The listing builds one solid part. Answer for the finished solid, in the listing's coordinates (mm). Face numbers are marked on the shaded views. A direction names the side the tool comes from. Round coordinates to 2 decimals unless told otherwise and drop trailing zeros. Order: outer loops, then holes, each group sorted by start corner. A loop starts at its lowest first (then second) coordinate and runs counter-clockwise, first axis right, second up. Notation, with made-up numbers: M -1.75,-37.5 L 23.25,-37.5 A24 cw 23.25,-26.5 Z; hole C 89.25,61.5 d4. An arc over 180 degrees is marked long. Write item = value, one per line. Start each with the question number.
(1) A cutting plane is placed at C-C, the plane x = 88.5. Determine the outline of the cut face in (y, z).
(2) For a pull along Z with two mould halves and no side action, classify the marked faces 1, 2, 3 and 4 as released by +Z, released by -Z, zero draft, split by the parting line, or undercut.
(3) A cutting plane is placed at B-B, the plane z = -24. Determine the outline of the cut face in (x, y), and give its area (3 significant figures).
(4) Straight lines are drawn through the part: probe 1 along Y at (x, z) = (230.5, -46); probe 2 along Z at (x, y) = (256, 197). For each, find the intervals that lie inside material, in ascending order. Write a range as from..to.
(5) A cutting plane is placed at A-A, the plane y = 224. Determine the outline of the cut face in (x, z), and give its area (3 significant figures).
(6) Which of the six approach directions +Z, -Z, +X, -X, +Y, -Y give full straight-line access (tool end or side, diameter ignored) to the marked faces 5 and 6?
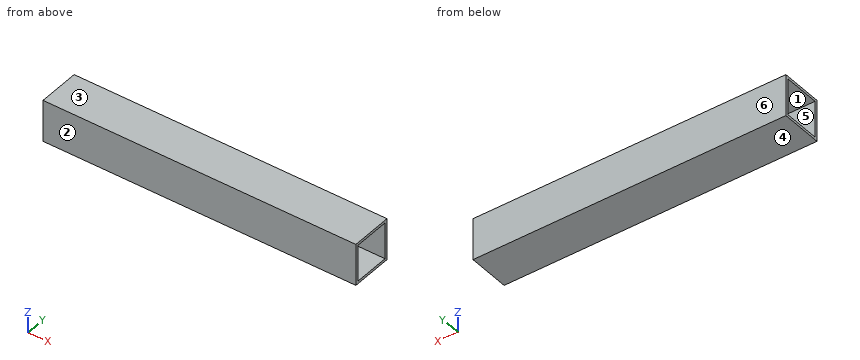
Solid Edge part; units mm, degrees
sketch "Sketch1" plane through (0, 0, 0) normal (1, 0, 0) x (0, 1, 0)
  line L0 (250, 0) -> (250, -80)
  line L1 (250, -80) -> (170, -80)
  line L2 (170, 0) -> (170, -80)
  line L3 (250, 0) -> (170, 0)
extrude "Protrusion1" add sketch "Sketch1" against normal up to vertex (250 mm away) and the other way up to vertex (350 mm away)
sketch "Sketch2" plane through (-250, 210, -40) normal (-1, 0, 0) x (0, -1, 0)
  line L0 (-35, 35) -> (-35, -35)
  line L1 (-35, -35) -> (35, -35)
  line L2 (35, -35) -> (35, 35)
  line L3 (35, 35) -> (-35, 35)
extrude "Cutout1" cut sketch "Sketch2" against normal through all
properties material "Fe360"
Reported:
q1.outline = M 170,-80 L 250,-80 L 250,0 L 170,0 Z; hole M 175,-75 L 245,-75 L 245,-5 L 175,-5 Z
q2.face_1 = undercut
q2.face_2 = zero draft
q2.face_3 = released by +Z
q2.face_4 = released by -Z
q3.outline = M -250,170 L 350,170 L 350,175 L -250,175 Z; M -250,245 L 350,245 L 350,250 L -250,250 Z
q3.area = 6,000 mm²
q4.probe_1 = 170..175, 245..250
q4.probe_2 = -80..-75, -5..0
q5.outline = M -250,-80 L 350,-80 L 350,-75 L -250,-75 Z; M -250,-5 L 350,-5 L 350,0 L -250,0 Z
q5.area = 6,000 mm²
q6.face_5 = +X, -X
q6.face_6 = +Z, -Z, +X, -X, +Y
